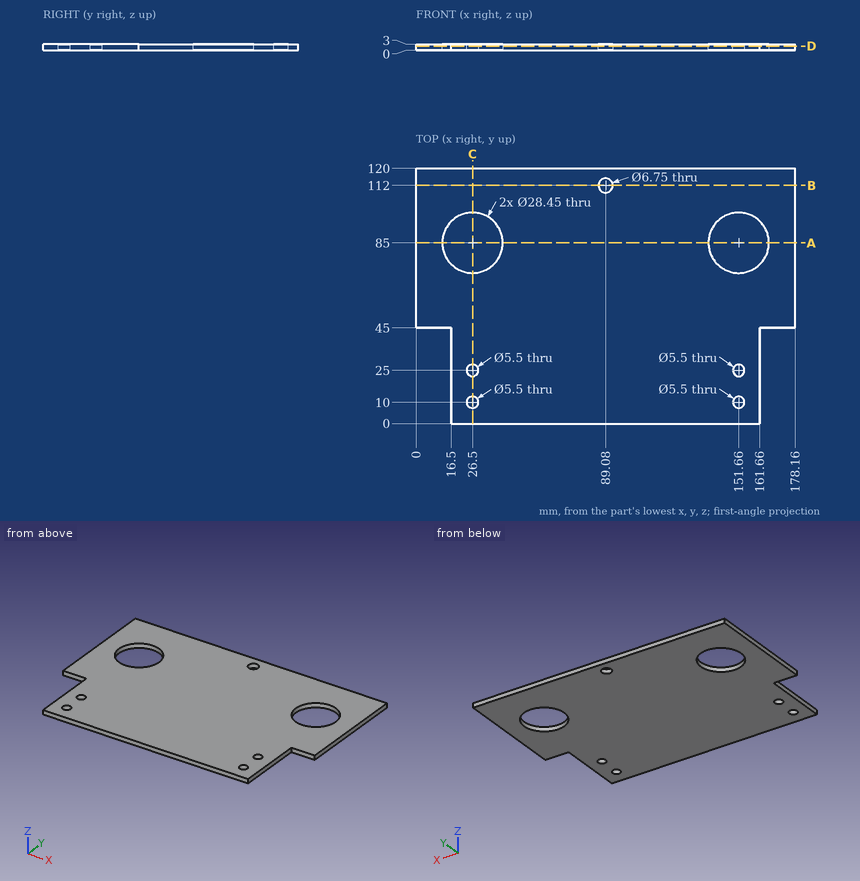
Source: three-view drawing plus pictorial views. Frame: mm from the lowest corner of the part. Round coordinates to 2 decimals unless told otherwise and drop trailing zeros. Loops run counter-clockwise (first coordinate to the right, second up) from the corner with the lowest first, then second, coordinate; pieces in that order, holes last.
Q1. Section A-A, the plane y = 85. Return loops of the section in (x, z) (3 decimals).
Q2. Ray query, line 1 (Y direction, x = 26.5, z = 2.35) (3 decimals); line 2 (X direction, y = 98, z = 1.25) (3 decimals); line 3 (Y direction, x = 89.5, z = 2.35). Return the intervals inside material, ascending.
Q3. First-contact query: P1, Ø5, axis at x = 26.5, y = 25, coming from the +Z side; P2, Ø6.5, axis at x = 26.5, y = 10, coming from the +Z side; P3, Ø1.5, axis at x = 169.5, z = 1, coming from the -Y side; P4, Ø1.5, axis at y = 25.5, z = 1, coming from the -X side. Flat tips, straight axial feed; report the tip coordinate or a pass-through.
Q4. Section D-D, the plane z = 2.05. Return loops of the section in (x, y) (3 decimals).
Q5. Section C-C, the plane x = 26.5. Return loops of the section in (y, z) (3 decimals), plus the area to 3 significant figures.
Q6. Section B-B, the plane y = 112. Return loops of the section in (x, z) (3 decimals), plus the area to 3 significant figures.
Solutions:
1. outline: (0, 0) - (12.275, 0) - (12.275, 3) - (0, 3) - close; (40.725, 0) - (137.435, 0) - (137.435, 3) - (40.725, 3) - close; (165.885, 0) - (178.16, 0) - (178.16, 3) - (165.885, 3) - close
2. line 1: y = 0 to 7.25, 12.75 to 22.25, 27.75 to 70.775, 99.225 to 120
2. line 2: x = 0 to 20.725, 32.275 to 145.885, 157.435 to 178.16
2. line 3: y = 0 to 108.65, 115.35 to 120
3. P1: passes through
3. P2: stops at z = 3
3. P3: stops at y = 45
3. P4: stops at x = 16.5
4. outline: (0, 45) - (16.5, 45) - (16.5, 0) - (161.66, 0) - (161.66, 45) - (178.16, 45) - (178.16, 120) - (0, 120) - close; hole circle Ø28.45 at (26.5, 85); hole circle Ø5.5 at (26.5, 10); hole circle Ø5.5 at (26.5, 25); hole circle Ø6.75 at (89.08, 112); hole circle Ø28.45 at (151.66, 85); hole circle Ø5.5 at (151.66, 10); hole circle Ø5.5 at (151.66, 25)
5. outline: (0, 0) - (7.25, 0) - (7.25, 3) - (0, 3) - close; (12.75, 0) - (22.25, 0) - (22.25, 3) - (12.75, 3) - close; (27.75, 0) - (70.775, 0) - (70.775, 3) - (27.75, 3) - close; (99.225, 0) - (120, 0) - (120, 3) - (99.225, 3) - close
5. area: 242 mm2
6. outline: (0, 0) - (85.705, 0) - (85.705, 3) - (0, 3) - close; (92.455, 0) - (178.16, 0) - (178.16, 3) - (92.455, 3) - close
6. area: 514 mm2
